Geometry check sheet. Reference: the model listing, model coordinates, mm. A direction names the side the tool comes from. Round coordinates to 2 decimals unless told otherwise and drop trailing zeros. Loops run counter-clockwise (first coordinate to the right, second up) from the corner with the lowest first, then second, coordinate; pieces in that order, holes last. Notation, with made-up numbers: M 70,-8 L 103,-8 A19 cw 103,18 Z; hole C -13.5,1 d6. An arc over 180 degrees is marked long. Write item = value, one per line.
from build123d import *

# Parameters (mm, degrees)
SKETCH1_R           = 19.304
BOSS_EXTRUDE1_DEPTH = 56.896
SKETCH2_R           = 6.35
BOSS_EXTRUDE2_DEPTH = 6.35
SKETCH3_R           = 1.575
CUT_EXTRUDE1_DEPTH  = 3.175
SKETCH4_R           = 1.5875
BOSS_EXTRUDE3_DEPTH = 8.89


with BuildPart() as part:
    # Sketch1 → Boss-Extrude1 (new body)
    with BuildSketch(Plane.XY):
        Circle(SKETCH1_R)
    extrude(amount=BOSS_EXTRUDE1_DEPTH)

    # Sketch2 → Boss-Extrude2 (add)
    with BuildSketch(Plane.XY.offset(56.896)):
        Circle(SKETCH2_R)
    extrude(amount=BOSS_EXTRUDE2_DEPTH)

    # Sketch3 → Cut-Extrude1 (cut)
    with BuildSketch(Plane.XY.offset(56.896)):
        with Locations((0, 12.3825)):
            Circle(SKETCH3_R)
        with Locations((0, -12.3825)):
            Circle(SKETCH3_R)
    extrude(amount=-CUT_EXTRUDE1_DEPTH, mode=Mode.SUBTRACT)

    # Sketch4 → Boss-Extrude3 (add)
    with BuildSketch(Plane.XY.offset(63.246)):
        Circle(SKETCH4_R)
    extrude(amount=BOSS_EXTRUDE3_DEPTH)


solid = part.part
(1) Sectioned sample at D-D on x = 9. Record the cut outline in (y, z).
Result set:
outline = M -17.08,0 L 17.08,0 L 17.08,56.9 L -17.08,56.9 Z
(2) Sectioned sample at B-B on y = 0. Record the cut outline in (x, z).
Result set:
outline = M -19.3,0 L 19.3,0 L 19.3,56.9 L 6.35,56.9 L 6.35,63.25 L 1.59,63.25 L 1.59,72.14 L -1.59,72.14 L -1.59,63.25 L -6.35,63.25 L -6.35,56.9 L -19.3,56.9 Z
(3) Depth check by flat-ended pin: pin 1 Ø1 at (y, z) = (-7, 44) entering from -X; pin 2 Ø1.6 at (x, y) = (-0.5, -12) entering from +Z; pin 3 Ø2 at (y, z) = (5.5, 56) entering from +X; pin 4 Ø1 at (y, z) = (14, 59) entering from -X. Enter the tip coordinate at first touch or a pass-through.
Result set:
pin_1 = -18.18
pin_2 = 53.72
pin_3 = 18.77
pin_4 = through
(4) Tool access check on faces 1 (the flat face through (0, 12, 53.721)), 2 (the flat face through (0, 0, 0)). Record the directions out of +Z, -Z, +X, -X, +Y, -Y that give a thin tool (end or side, any length) a straight path to the whole face; none if there is none.
Result set:
face_1 = +Z
face_2 = -Z, +X, -X, +Y, -Y
(5) Sectioned sample at A-A on x = 0. Record the cut outline in (y, z), then the cut area to 3 significant figures.
Result set:
outline = M -19.3,0 L 19.3,0 L 19.3,56.9 L 13.96,56.9 L 13.96,53.72 L 10.81,53.72 L 10.81,56.9 L 6.35,56.9 L 6.35,63.25 L 1.59,63.25 L 1.59,72.14 L -1.59,72.14 L -1.59,63.25 L -6.35,63.25 L -6.35,56.9 L -10.81,56.9 L -10.81,53.72 L -13.96,53.72 L -13.96,56.9 L -19.3,56.9 Z
area = 2,290 mm2
(6) Material ranges on line 1 along Y through (x, z) = (0, 55.35); line 2 along Z through (x, y) = (9, -13); line 3 along Y through (x, z) = (-0.5, 55.5), recorded low to high. Write a range as from..to.
Result set:
line_1 = -19.3..-13.96, -10.81..10.81, 13.96..19.3
line_2 = 0..56.9
line_3 = -19.3..-13.88, -10.89..10.89, 13.88..19.3
(7) Sectioned sample at C-C on z = 18. Record the cut outline in (x, y).
Result set:
outline = C 0,0 d38.61
(8) Release check for a two-part mould opening along X. For faces 3 (the flat face through (-5, 5, 56.896)), 4 (the cylindrical face through (-15.319, -11.746, 28.05)), 5 (the flat face through (0, -12, 53.721)) record: released by +X, released by -X, zero draft, split by the parting line, or undercut.
Result set:
face_3 = zero draft
face_4 = split by the parting line
face_5 = undercut
